Verification items for the finished model (mm, model axes). Give positions to 0.01 mm unless a question says otherwise; leave off trailing zeros. Order: outer loops, then holes, each group sorted by start corner. A loop starts at its lowest first (then second) coordinate and runs counter-clockwise, first axis right, second up. Notation, with made-up numbers: (29.25, 71.5) -> (58.25, 71.5) arc R29 cw to (58.25, 91.5) -> close; hole circle Ø2 at (-37.75, 37). An arc over 180 degrees is marked (long way). One line per question, with ' | ' between items. Start each with the question number.
Q1. Section check D-D on y = -3.85. Give the number of separate pieces and of enclosed holes in the cut face, plus the area to 3 significant figures.
Q2. Material ranges on probe 1 along Z at (x, y) = (69.5, -4.8); probe 2 along Z at (x, y) = (0, -1.2); probe 3 along X at (y, z) = (-0.8, 55.5), recorded low to high. Write a range as [from, to].
Q3. Section check C-C on z = 57.5. Record the cut outline in (x, y).
Q4. Go/stop test with flat-tipped pins: pin 1 (1.8 mm diameter, centred on x = -69, y = -1.5, fed in from -Z); pin 2 (2 mm diameter, centred on y = -3, z = 29.5, fed in from +X). Record where each tip stops, or that it passes through.
Q5. Section check B-B on x = 0. Record the cut outline in (y, z).
Q6. Section check A-A on z = 13. Record the cut outline in (x, y), plus the area to 3 significant figures.
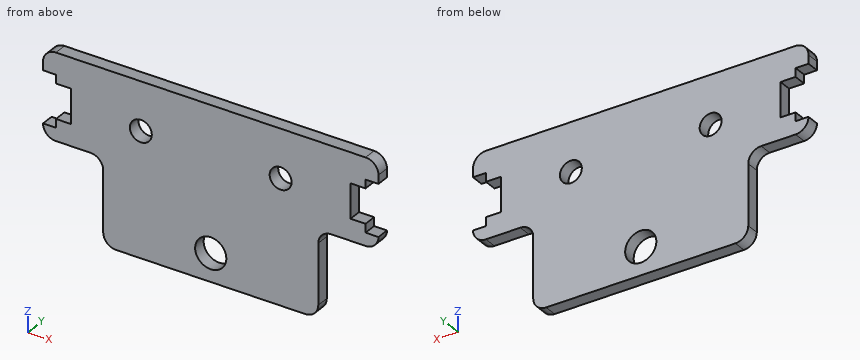
from build123d import *
from build123d import SkipClean  # not in build123d's __all__

# Parameters (mm, degrees)
F1_DEPTH = 6
F2_R     = 5.1
F3_DEPTH = 25
F5_DEPTH = 25
F6_R     = 5.99999
F8_R     = 6


# Not quite as in the source:
# - a fillet or chamfer is up to 0.001 mm smaller than in the source, because OpenCascade refuses the exact size


with BuildPart() as f1:
    # F0 (on Front) → F1 (new body)
    with BuildSketch(Plane.XZ):
        Polygon((-50, 0), (0, 0), (0, 80), (-78, 80), (-78, 70), (-72, 70), (-72, 66), (-65, 66), (-65, 50), (-72, 50), (-72, 46), (-78, 46), (-78, 40), (-50, 40), align=None)
    extrude(amount=F1_DEPTH)

    # F2 (on face) → F3 (cut)
    with BuildSketch(Plane.XZ.offset(6)):
        with Locations((-32.5, 57.5)):
            Circle(F2_R)
    extrude(amount=-F3_DEPTH, mode=Mode.SUBTRACT)

    # F4 (on face) → F5 (cut)
    with BuildSketch(Plane.XZ.offset(6)):
        with BuildLine():
            Line((0, 5.75), (0, 20.25))
            ThreePointArc((0, 20.25), (-7.25, 13), (0, 5.75))
        make_face()
    extrude(amount=-F5_DEPTH, mode=Mode.SUBTRACT)

    # F6 (radius 6 in the source; OpenCascade refuses exactly that, so slightly less here)
    f6_edges = [f1.edges().sort_by_distance(p)[0] for p in [
        (-78, -3, 80),
        (-78, -3, 40),
        (-50, -3, 0),
    ]]
    fillet(f6_edges, radius=F6_R)

    # F7: F1 across face


with BuildPart() as f1_1:
    add(f1.part, clean=False)
    with SkipClean():  # cleaning this boolean's faces spoils the solid; the shape is the same uncleaned
        add(f1.part.mirror(Plane(origin=(0, -3, 50.125), x_dir=(0, 1, 0), z_dir=(1, 0, 0))), clean=False)

    # F8
    f8_edges = [f1_1.edges().sort_by_distance(p)[0] for p in [
        (-50, -3, 40),
        (50, -3, 40),
    ]]
    fillet(f8_edges, radius=F8_R)


solid = f1_1.part
Filled in:
1) separate pieces: 1 | enclosed holes: 3 | area: 9,370 mm²
2) probe 1: [40, 50], [66, 80] | probe 2: [0, 5.75], [20.25, 80] | probe 3: [-65, -37.19], [-27.81, 27.81], [37.19, 65]
3) outline: (-65, -6) -> (-37.6, -6) -> (-37.6, 0) -> (-65, 0) -> close; (-27.4, -6) -> (27.4, -6) -> (27.4, 0) -> (-27.4, 0) -> close; (37.6, -6) -> (65, -6) -> (65, 0) -> (37.6, 0) -> close
4) pin 1: z = 40 | pin 2: x = 50
5) outline: (-6, 0) -> (0, 0) -> (0, 5.75) -> (-6, 5.75) -> close; (-6, 20.25) -> (0, 20.25) -> (0, 80) -> (-6, 80) -> close
6) outline: (-50, -6) -> (-7.25, -6) -> (-7.25, 0) -> (-50, 0) -> close; (7.25, -6) -> (50, -6) -> (50, 0) -> (7.25, 0) -> close | area: 513 mm²
